Geometry: final body of the model. Coordinates: model frame, mm. A direction names the side the tool comes from. Give positions to 0.01 mm unless a question says otherwise; leave off trailing zeros. Write each loop counter-clockwise with the first axis right and the second up, starting at its lowest first coordinate (ties: lowest second). Pieces come first, ordered by that corner, then holes. Notation, with made-up numbers: (41, 86.25) -> (91, 86.25) arc R25 ccw to (91, 108.25) -> close; hole circle Ø8 at (3, 66). An arc over 180 degrees is marked (long way). Answer as a JSON object with one key per item and string values.
from build123d import *

# Parameters (mm, degrees)
SKETCH_1_W      = 7
SKETCH_1_H      = 6
EXTRUDE_1_DEPTH = 2.5
SKETCH_2_W      = 7
SKETCH_2_H      = 2.5
EXTRUDE_2_DEPTH = 2.5
SKETCH_3_W      = 7
SKETCH_3_H      = 1
EXTRUDE_3_DEPTH = 1
SKETCH_4_W      = 5
SKETCH_4_H      = 1
EXTRUDE_4_DEPTH = 4.5
SKETCH_5_W      = 4
SKETCH_5_H      = 1
EXTRUDE_5_DEPTH = 10
CHAMFER_1_SIZE  = 1


with BuildPart() as part:
    # 스케치1 → 보스-돌출1 (new body)
    with BuildSketch(Plane.XY):
        Rectangle(SKETCH_1_W, SKETCH_1_H)
    extrude(amount=EXTRUDE_1_DEPTH)

    # 스케치2 → 보스-돌출2 (add)
    with BuildSketch(Plane.XY.offset(2.5)):
        Rectangle(SKETCH_2_W, SKETCH_2_H)
    extrude(amount=EXTRUDE_2_DEPTH)

    # 스케치3 → 보스-돌출3 (add)
    with BuildSketch(Plane.XY.offset(5)):
        Rectangle(SKETCH_3_W, SKETCH_3_H)
    extrude(amount=EXTRUDE_3_DEPTH)

    # 스케치4 → 보스-돌출4 (add)
    with BuildSketch(Plane.XY.offset(6)):
        Rectangle(SKETCH_4_W, SKETCH_4_H)
    extrude(amount=EXTRUDE_4_DEPTH)

    # 스케치5 → 보스-돌출5 (add)
    with BuildSketch(Plane.XY.offset(10.5)):
        Rectangle(SKETCH_5_W, SKETCH_5_H)
    extrude(amount=EXTRUDE_5_DEPTH)

    # 모따기1
    chamfer_1_edges = [part.edges().sort_by_distance(p)[0] for p in [
        (3.5, 0, 6),
        (-3.5, 0, 6),
    ]]
    chamfer(chamfer_1_edges, length=CHAMFER_1_SIZE - 0.0001)  # a hair under: the kernel refuses the full size


solid = part.part
Q1. Set-up query: faces 1 (the flat face through (0, 0.5, 13)), 2 (the flat face through (-2, 0, 15)), 3 (the flat face through (2.5, 0, 8)), 4 (the flat face through (0, -2, 2.5)). Return all of +Z, -Z, +X, -X, +Y, -Y with unobstructed straight access to the full face (end or side cutting, diameter ignored); none if empty.
Values:
{"face 1": "+Z, +X, -X, +Y", "face 2": "+Z, -X, +Y, -Y", "face 3": "+Z, +X, +Y, -Y", "face 4": "+Z, +X, -X, -Y"}
Q2. Cut plane A-A (x = 0.75). Return the cut outline in (y, z), and give its area (4 significant figures).
Values:
{"outline": "(-3, 0) -> (3, 0) -> (3, 2.5) -> (1.25, 2.5) -> (1.25, 5) -> (0.5, 5) -> (0.5, 20.5) -> (-0.5, 20.5) -> (-0.5, 5) -> (-1.25, 5) -> (-1.25, 2.5) -> (-3, 2.5) -> close", "area": "36.75 mm²"}
Q3. Cut plane C-C (y = -2.3). Return the cut outline in (x, z), and give its area (3 significant figures).
Values:
{"outline": "(-3.5, 0) -> (3.5, 0) -> (3.5, 2.5) -> (-3.5, 2.5) -> close", "area": "17.5 mm²"}
Q4. Cut plane B-B (z = 3.75). Return the cut outline in (x, y), and give its area (3 significant figures).
Values:
{"outline": "(-3.5, -1.25) -> (3.5, -1.25) -> (3.5, 1.25) -> (-3.5, 1.25) -> close", "area": "17.5 mm²"}
Q5. Material intervals for L1, parallel to Y at x = -1, z = 19.75; L2, parallel to Z at x = 2.25, y = -0.25; L3, parallel to Y at x = -3, z = 3.25, sorted ascending. Write a range as from..to.
Values:
{"L1": "-0.5..0.5", "L2": "0..10.5", "L3": "-1.25..1.25"}
Q6. Mould query, pull axis Y, two halves, no side actions, for faces 5 (the flat face through (0, 1.25, 4)), 6 (the flat face through (0, -3, 1)), 7 (the flat face through (-2.5, 0, 8)). Classes: pulls with the +Y half, pulls with the -Y half, needs draft (parallel to the pull), parting line crosses it, or undercut.
Values:
{"face 5": "pulls with the +Y half", "face 6": "pulls with the -Y half", "face 7": "needs draft"}
Q7. First-contact query: P1, Ø0.8, axis at y = 0, z = 15, coming from the +X side; P2, Ø3, axis at x = 2.5, z = 10.5, coming from the +Y side; P3, Ø0.9, axis at x = 0, y = 2, coming from the +Z side. Flat tips, straight axial feed; report the tip coordinate or a pass-through.
Values:
{"P1": "x = 2", "P2": "y = 0.5", "P3": "z = 2.5"}
